Input: part model. Units: mm. Frame: model coordinates. Face numbers are marked on the shaded views. A direction names the side the tool comes from. Coordinates: 2 decimals unless noted, no trailing zeros. Write each loop counter-clockwise with the first axis right and the second up, starting at its lowest first coordinate (ties: lowest second). Pieces come first, ordered by that corner, then holes. Notation, with made-up numbers: (-5.5, -25.75) -> (42.5, -25.75) arc R20 ccw to (42.5, -16.75) -> close; hole circle Ø4 at (-14.5, 50.25). An arc over 180 degrees is marked (long way). One line per question, with ' | ' between items. Start each with the question number.
```python
from build123d import *

# Parameters (mm, degrees)
F0_W      = 50
F0_H      = 50
F1_DEPTH  = 4
F2_W      = 44
F2_H      = 44
F3_DEPTH  = 3
F4_R      = 3
F5_DEPTH  = 25
F6_R      = 5
F6_R_2    = 3
F7_DEPTH  = 5
F8_R      = 16
F9_DEPTH  = 5
F10_R     = 8
F11_DEPTH = 25
F12_R     = 3


# Not quite as in the source:
# - a feature names something its author has since deleted; it is built from what else it names


with BuildPart() as f1:
    # F0 (on Front) → F1 (new body)
    with BuildSketch(Plane.XZ):
        Rectangle(F0_W, F0_H)
    extrude(amount=-F1_DEPTH)

    # F2 (on face) → F3 (join)
    with BuildSketch(Plane(origin=(0, 4, 0), x_dir=(-1, 0, 0), z_dir=(0, 1, 0))):
        Rectangle(F2_W, F2_H)
    extrude(amount=F3_DEPTH)

    # F4 (on face) → F5 (cut)
    with BuildSketch(Plane(origin=(0, 7, 0), x_dir=(-1, 0, 0), z_dir=(0, 1, 0))):
        with Locations((-16.5, 16.5)):
            Circle(F4_R)
        with Locations((16.5, 16.5)):
            Circle(F4_R)
        with Locations((16.5, -16.5)):
            Circle(F4_R)
        with Locations((-16.5, -16.5)):
            Circle(F4_R)
    extrude(amount=-F5_DEPTH, mode=Mode.SUBTRACT)

    # F6 (on face) → F7 (cut)
    with BuildSketch(Plane.XZ):
        with Locations((-16.5, 16.5)):
            Circle(F6_R)
        with Locations((-16.5, 16.5)):
            Circle(F6_R_2, mode=Mode.SUBTRACT)
        with Locations((16.5, 16.5)):
            Circle(F6_R)
        with Locations((16.5, 16.5)):
            Circle(F6_R_2, mode=Mode.SUBTRACT)
        with Locations((16.5, -16.5)):
            Circle(F6_R)
        with Locations((16.5, -16.5)):
            Circle(F6_R_2, mode=Mode.SUBTRACT)
        with Locations((-16.5, -16.5)):
            Circle(F6_R)
        with Locations((-16.5, -16.5)):
            Circle(F6_R_2, mode=Mode.SUBTRACT)
    extrude(amount=-F7_DEPTH, mode=Mode.SUBTRACT)

    # F8 (on face) → F9 (cut)
    with BuildSketch(Plane(origin=(0, 7, 0), x_dir=(-1, 0, 0), z_dir=(0, 1, 0))):
        Circle(F8_R)
    extrude(amount=-F9_DEPTH, mode=Mode.SUBTRACT)

    # F10 (on face) → F11 (cut)
    with BuildSketch(Plane(origin=(0, 2, 0), x_dir=(-1, 0, 0), z_dir=(0, 1, 0))):
        Circle(F10_R)
    extrude(amount=-F11_DEPTH, mode=Mode.SUBTRACT)

    # F12
    f12_edges = [f1.edges().sort_by_distance(p)[0] for p in [
        (-22, 5.5, 22),
        (-22, 5.5, -22),
        (22, 5.5, -22),
        (22, 5.5, 22),
    ]]
    fillet(f12_edges, radius=F12_R)


solid = f1.part
```
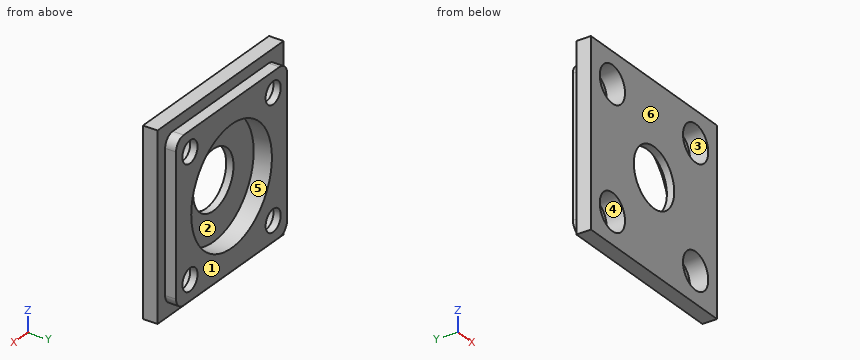
1) Access query for the marked faces 4, 5 and 6. Directions: +Z, -Z, +X, -X, +Y, -Y. A direction counts if a zero-diameter tool reaches every point of the face in a straight line with its end or side. Return the directions, or none.
2) Section D-D, the plane z = -9. Return loops of the section in (x, y).
3) Ray query, line 1 (Z direction, x = -16.5, y = 6.65); line 2 (Z direction, x = 16.5, y = 2.2); line 3 (X direction, y = 6, z = 19). Return the intervals inside material, ascending.
4) First-contact query: P1, Ø1.5, axis at x = -5, y = 5, coming from the -Z side; P2, Ø2, axis at y = 5.5, z = 15, coming from the +X side; P3, Ø0.9, axis at y = 5, z = 0, coming from the -X side. Flat tips, straight axial feed; report the tip coordinate or a pass-through.
5) Section C-C, the plane x = 0. Return loops of the section in (y, z), then the cut area to 3 significant figures.
6) Pull-direction query (X, two-part tool) for the marked faces 1, 2 and 3; classes: released by +X, released by -X, zero draft, split by the parting line, or undercut.
7) Section A-A, the plane y = 3. Return loops of the section in (x, z), then the cut area to 3 significant figures.
8) Section B-B, the plane z = 0. Return loops of the section in (x, y), then the cut area to 3 significant figures.
Answer block:
1) face 4: -Y | face 5: +Y | face 6: +Z, -Z, +X, -X, -Y
2) outline: (-25, 0) -> (25, 0) -> (25, 4) -> (22, 4) -> (22, 7) -> (13.23, 7) -> (13.23, 2) -> (-13.23, 2) -> (-13.23, 7) -> (-22, 7) -> (-22, 4) -> (-25, 4) -> close
3) line 1: z = -22 to -19.5, -13.5 to 13.5, 19.5 to 22 | line 2: z = -25 to -21.5, -11.5 to 11.5, 21.5 to 25 | line 3: x = -22 to -18.16, -14.84 to 14.84, 18.16 to 22
4) P1: stops at z = -22 | P2: stops at x = 22 | P3: stops at x = -22
5) outline: (0, -25) -> (4, -25) -> (4, -22) -> (7, -22) -> (7, -16) -> (2, -16) -> (2, -8) -> (0, -8) -> close; (0, 8) -> (2, 8) -> (2, 16) -> (7, 16) -> (7, 22) -> (4, 22) -> (4, 25) -> (0, 25) -> close | area: 140 mm2
6) face 1: zero draft | face 2: undercut | face 3: undercut
7) outline: (-25, -25) -> (25, -25) -> (25, 25) -> (-25, 25) -> close; hole circle Ø10 at (-16.5, -16.5); hole circle Ø10 at (-16.5, 16.5); hole circle Ø32 at (0, 0); hole circle Ø10 at (16.5, -16.5); hole circle Ø10 at (16.5, 16.5) | area: 1,380 mm2
8) outline: (-25, 0) -> (-8, 0) -> (-8, 2) -> (-16, 2) -> (-16, 7) -> (-22, 7) -> (-22, 4) -> (-25, 4) -> close; (8, 0) -> (25, 0) -> (25, 4) -> (22, 4) -> (22, 7) -> (16, 7) -> (16, 2) -> (8, 2) -> close | area: 140 mm2
